from build123d import *

# Parameters (mm, degrees)
SKETCH1_R           = 2.325
SKETCH1_R_2         = 3
BOSS_EXTRUDE1_DEPTH = 3
BOSS_EXTRUDE2_START = -1
SKETCH1_3_R         = 4.325
SKETCH1_3_R_2       = 2.325
BOSS_EXTRUDE2_DEPTH = 1


with BuildPart() as part:
    # Sketch1 → Boss-Extrude1 (new body)
    with BuildSketch(Plane.XY):
        with BuildLine():
            Line((-4.997151532, 19.83125), (-4.322536076, -0.14596875))
            ThreePointArc((-4.322536076, -0.14596875), (0, -4.325), (4.322536076, -0.14596875))
            Line((4.322536076, -0.14596875), (4.997151532, 19.83125))
            ThreePointArc((4.997151532, 19.83125), (0, 25), (-4.997151532, 19.83125))
        make_face()
        Circle(SKETCH1_R, mode=Mode.SUBTRACT)
        with Locations((0, 20)):
            Circle(SKETCH1_R_2, mode=Mode.SUBTRACT)
    extrude(amount=BOSS_EXTRUDE1_DEPTH)

    # Sketch1<3> → Boss-Extrude2 (add)
    with BuildSketch(Plane.XY.offset(BOSS_EXTRUDE2_START)):
        with Locations(Location((0, 0, 0), (0, 0, 181.934099854))):
            Circle(SKETCH1_3_R)
        Circle(SKETCH1_3_R_2, mode=Mode.SUBTRACT)
    extrude(amount=BOSS_EXTRUDE2_DEPTH)


solid = part.part
Can you work these out from the model? Positions are in its coordinate system, mm. Coordinates: 2 decimals unless noted, no trailing zeros. Loops run counter-clockwise (first coordinate to the right, second up) from the corner with the lowest first, then second, coordinate; pieces in that order, holes last. Notation, with made-up numbers: (66, 69.25) - (103, 69.25) arc R7 ccw to (103, 77.25) - close; hole circle Ø10 at (2.5, 41). An arc over 180 degrees is marked (long way). Put each result on its own line as item: value. Start each with the question number.
Item 1: If we mould it in two halves opening along Y, with no side actions, what happens to faces 1 (the face through (1.25, 1.96, 0.97)), 2 (the face through (0, 13, 0))? For each: +Y half, -Y half, draft (parallel to the pull), parting line (faces both ways), or undercut.
Item 2: For pin 1 (2 mm diameter, centred on x = 4, y = 21, fed in from -Z); pin 2 (2 mm diameter, centred on y = -0.5, z = 0, fed in from +X); pin 3 (1 mm diameter, centred on y = 17.5, z = 0.5, fed in from -X); pin 4 (3.5 mm diameter, centred on x = 0, y = 20, fed in from +Z), each with a flat end and sliding along its axis, tell me the tip position at first contact or that it passes through.
Item 3: Suppose I cut it at A-A (x = 0). Please give me the cut outline in (y, z) (3 decimals).
Item 4: Suppose I cut it at B-B (y = 19.5). Please give me the cut outline in (x, z), and give its area (3 significant figures).
Item 5: If I drill on line 1 along Y through (x, z) = (0, 1.4) (3 decimals); line 2 along Y through (x, z) = (0, -0.8) (3 decimals); line 3 along Y through (x, z) = (-1, 1.6), over which ranges is the centre line in solid material (lowest first)?
Item 6: Suppose I cut it at C-C (z = 2.4). Please give me the cut outline in (x, y) (3 decimals), and give its area (3 significant figures).
Item 7: Suppose I cut it at D-D (z = -0.65). Please give me the cut outline in (x, y) (3 decimals).
Here are the results:
1. face 1: undercut
1. face 2: draft
2. pin 1: z = 0
2. pin 2: x = 4.34
2. pin 3: x = -4.94
2. pin 4: through
3. outline: (-4.325, -1) - (-2.325, -1) - (-2.325, 3) - (-4.325, 3) - close; (2.325, -1) - (4.325, -1) - (4.325, 0) - (17, 0) - (17, 3) - (2.325, 3) - close; (23, 0) - (25, 0) - (25, 3) - (23, 3) - close
4. outline: (-4.99, 0) - (-2.96, 0) - (-2.96, 3) - (-4.99, 3) - close; (2.96, 0) - (4.99, 0) - (4.99, 3) - (2.96, 3) - close
4. area: 12.2 mm²
5. line 1: -4.325 to -2.325, 2.325 to 17, 23 to 25
5. line 2: -4.325 to -2.325, 2.325 to 4.325
5. line 3: -4.21 to -2.1, 2.1 to 17.17, 22.83 to 24.9
6. outline: (-4.997, 19.831) - (-4.323, -0.146) arc R4.325 ccw to (4.323, -0.146) - (4.997, 19.831) arc R5 ccw (long way) to start; hole circle Ø6 at (0, 20); hole circle Ø4.65 at (0, 0)
6. area: 210 mm²
7. outline: circle Ø8.65 at (0, 0); hole circle Ø4.65 at (0, 0)
